Design review of the part built by this model. Coordinates are the model's own, in mm. Give positions to 0.01 mm unless a question says otherwise; leave off trailing zeros. Loops run counter-clockwise (first coordinate to the right, second up) from the corner with the lowest first, then second, coordinate; pieces in that order, holes last.
from build123d import *

# Parameters (mm, degrees)
CYLINDER019_R     = 1.5
CYLINDER019_DEPTH = 10
ARRAY_X_COUNT     = 2
ARRAY_X_PITCH     = 24
ARRAY_Y_COUNT     = 2
ARRAY_Y_PITCH     = 24
CYLINDER014_R     = 10
CYLINDER014_DEPTH = 6
CYLINDER018_R     = 20
CYLINDER018_DEPTH = 6
FILLET_R          = 1


with BuildPart() as bolt_hole_array:
    # Cylinder019 → Cylinder019 (new body)
    with BuildSketch(Plane.XY):
        Circle(CYLINDER019_R)
    extrude(amount=CYLINDER019_DEPTH)

    # Array X: bolt hole array ×2


with BuildPart() as bolt_hole_array_1:
    add(bolt_hole_array.part)
    with Locations(*[(i * ARRAY_X_PITCH, 0, 0) for i in range(1, ARRAY_X_COUNT)]):
        add(bolt_hole_array.part)

    # Array Y: bolt hole array ×2


with BuildPart() as bolt_hole_array_2:
    add(bolt_hole_array_1.part)
    with Locations(*[(0, i * ARRAY_Y_PITCH, 0) for i in range(1, ARRAY_Y_COUNT)]):
        add(bolt_hole_array_1.part)


with BuildPart() as bolt_hole_array_3:
    # Array placement: moved
    add(bolt_hole_array_2.part.moved(Location((-12, -12, 0))))


with BuildPart() as hole_fusion:
    # Cylinder014 → Cylinder014 (new body)
    with BuildSketch(Plane.XY):
        Circle(CYLINDER014_R)
    extrude(amount=CYLINDER014_DEPTH)

    # Fusion003: union bolt hole array
    add(bolt_hole_array_3.part)


with BuildPart() as fillet_body:
    # Cylinder018 → Cylinder018 (new body)
    with BuildSketch(Plane.XY):
        Circle(CYLINDER018_R)
    extrude(amount=CYLINDER018_DEPTH)

    # Cut003: cut hole fusion
    add(hole_fusion.part, mode=Mode.SUBTRACT)

    # Fillet
    fillet_edges = [fillet_body.edges().sort_by_distance(p)[0] for p in [
        (-20, 0, 6),
        (-20, 0, 0),
        (-10, 0, 6),
    ]]
    fillet(fillet_edges, radius=FILLET_R)


solid = fillet_body.part
Q1. Take a section at A-A (x = 0). Give the boundary of the cut face in (y, z), plus the area to 3 significant figures.
Results:
outline: (-20, 1) arc R1 ccw to (-19, 0) - (-10, 0) - (-10, 5) arc R1 ccw to (-11, 6) - (-19, 6) arc R1 ccw to (-20, 5) - close; (10, 0) - (19, 0) arc R1 ccw to (20, 1) - (20, 5) arc R1 ccw to (19, 6) - (11, 6) arc R1 ccw to (10, 5) - close
area: 119 mm2
Q2. Take a section at D-D (y = 12). Give the number of separate pieces and of enclosed holes in the cut face, plus the area to 3 significant figures.
Results:
separate pieces: 3
enclosed holes: 0
area: 155 mm2
Q3. Insertion check: pin 1 (1.8 mm diameter, centred on x = 12, y = -12, fed in from -Z); pin 2 (2 mm diameter, centred on y = 2.5, z = 4.5, fed in from +X); pin 3 (10 mm diameter, centred on x = 0, y = -8.5, fed in from -Z); pin 4 (1 mm diameter, centred on x = 10, z = 3.5, fed in from -Y). Each pin has a flat end and moves straight along its axis. Give the tip position at first contact, or say it passes through.
Results:
pin 1: passes through
pin 2: stops at x = 19.94
pin 3: stops at z = 0
pin 4: stops at y = -17.6
Q4. Take a section at C-C (z = 2.45). Give the boundary of the cut face in (x, y), plus the area to 3 significant figures.
Results:
outline: circle Ø40 at (0, 0); hole circle Ø3 at (-12, -12); hole circle Ø3 at (-12, 12); hole circle Ø20 at (0, 0); hole circle Ø3 at (12, -12); hole circle Ø3 at (12, 12)
area: 914 mm2
Q5. Draft analysis for pull direction X (two halves, no side actions). For faces 1 (the face through (-2.17, -9.76, 2.46)), 2 (the face through (8, -8, 0)), 3 (the face through (-4.336, -19.524, 2.972)), state which applies: pulls with the +X half, pulls with the -X half, needs draft (parallel to the pull), parting line crosses it, or undercut.
Results:
face 1: undercut
face 2: needs draft
face 3: parting line crosses it
Q6. Wall thickness on line 1 (X direction, y = 12, z = 3.05); line 2 (Y direction, x = 12.5, z = 4.15): over which ranges is each line inside the solid? List them lowest first.
Results:
line 1: x = -16 to -13.5, -10.5 to 10.5, 13.5 to 16
line 2: y = -15.61 to -13.41, -10.59 to 10.59, 13.41 to 15.61
